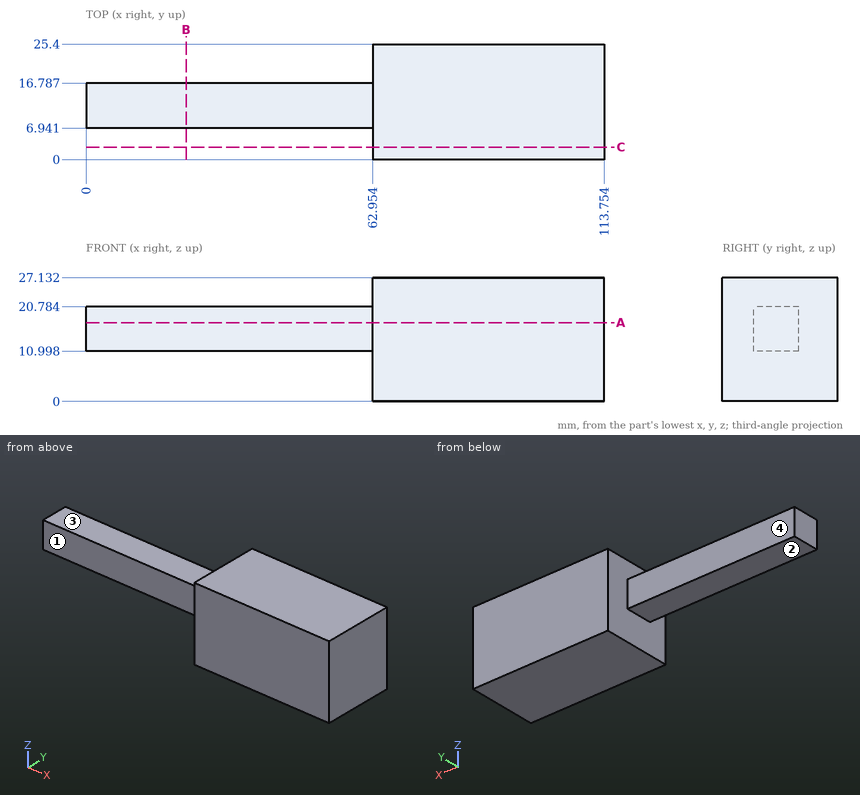
Here's the drawing with two shaded views (mm, measured from the low corner). I have some questions. A direction names the side the tool comes from. Give positions to 0.01 mm unless a question says otherwise; leave off trailing zeros. Loops run counter-clockwise (first coordinate to the right, second up) from the corner with the lowest first, then second, coordinate; pieces in that order, holes last. Notation, with made-up numbers: (-33.5, -12.75) -> (-9.5, -12.75) arc R11 cw to (-9.5, 1.25) -> close; hole circle Ø9 at (21, -7). An arc over 180 degrees is marked (long way). Use one line per item in the form item = value.
1) I need wall thicknesses on line 1 along X through (y, z) = (19.5, 6.25); line 2 along Z through (x, y) = (11, 9.75) (1 decimal); line 3 along Y through (x, z) = (56, 17). Which ranges of each line are inside material? Lowest first, please.
Answers:
line_1 = 62.95 to 113.75
line_2 = 11 to 20.8
line_3 = 6.94 to 16.79
2) For the marked faces 1, 2, 3 and 4, which set-ups out of +Z, -Z, +X, -X, +Y, -Y let a thin tool reach every point of the face, with its end or its side?
Answers:
face_1 = +Z, -Z, -X, -Y
face_2 = -Z, -X, +Y, -Y
face_3 = +Z, -X, +Y, -Y
face_4 = +Z, -Z, -X, +Y
3) If we section it at B-B (x = 22): Please give me the cut outline in (y, z) (1 decimal).
Answers:
outline = (6.9, 11) -> (16.8, 11) -> (16.8, 20.8) -> (6.9, 20.8) -> close
4) If we section it at C-C (y = 2.75): Please give me the cut outline in (x, z).
Answers:
outline = (62.95, 0) -> (113.75, 0) -> (113.75, 27.13) -> (62.95, 27.13) -> close
5) If we section it at A-A (z = 17.25): Please give me the cut outline in (x, y), plus the area to 3 significant figures.
Answers:
outline = (0, 6.94) -> (62.95, 6.94) -> (62.95, 0) -> (113.75, 0) -> (113.75, 25.4) -> (62.95, 25.4) -> (62.95, 16.79) -> (0, 16.79) -> close
area = 1,910 mm²
6) Will these pins go through, and if not, where does the flat tip stop? pin 1 (11 mm diameter, centred on x = 39.5, z = 16.5, fed in from -Y); pin 2 (10 mm diameter, centred on x = 56, y = 18.5, fed in from -Z); pin 3 (3 mm diameter, centred on x = 76.5, z = 6, fed in from -Y); pin 4 (3 mm diameter, centred on x = 42, y = 10.5, fed in from +Z).
Answers:
pin_1 = 6.94
pin_2 = 11
pin_3 = 0
pin_4 = 20.78
